Study the drawing (mm; zero at the part's minimum x, y, z) and answer. Give positions to 0.01 mm unless a question says otherwise; leave off trailing zeros. Write each loop counter-clockwise with the first axis right and the second up, starting at its lowest first coordinate (ties: lowest second). Pieces come first, ordered by that corner, then holes.
1) Find section C-C (z = 5). Determine the outline of the cut face in (x, y), plus the area to 3 significant figures.
2) Find section A-A (y = 10). Determine the outline of the cut face in (x, z), plus the area to 3 significant figures.
3) Straight lines are drawn through the part: probe 1 along Y at (x, z) = (10, 21); probe 2 along Z at (x, y) = (8.5, 12.5); probe 3 along X at (y, z) = (7.5, 43). For each, find the intervals that lie inside material, in ascending order.
4) Given pin 1 Ø8 at (x, z) = (6.5, 57) entering from +Y; pin 2 Ø6 at (y, z) = (12, 23) entering from +X; pin 3 Ø5.5 at (x, y) = (10, 10) entering from -Z, each flat-ended and moving along its own axis, determine where each tip first touches the part or whether it passes through.
5) Find section D-D (z = 15). Determine the outline of the cut face in (x, y), plus the area to 3 significant figures.
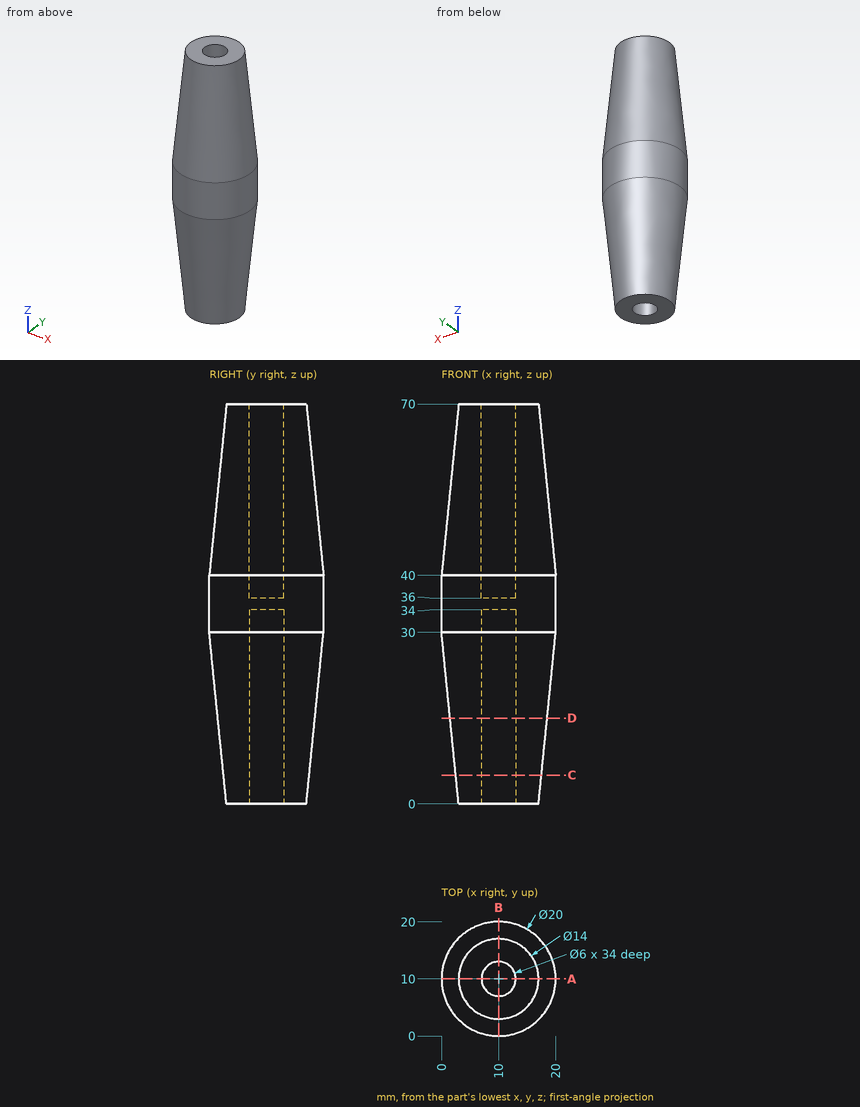
Results:
1. outline: circle Ø15 at (10, 10); hole circle Ø6 at (10, 10)
1. area: 148 mm2
2. outline: (0, 30) - (3, 0) - (7, 0) - (7, 34) - (13, 34) - (13, 0) - (17, 0) - (20, 30) - (20, 40) - (17, 70) - (13, 70) - (13, 36) - (7, 36) - (7, 70) - (3, 70) - (0, 40) - close
2. area: 812 mm2
3. probe 1: y = 0.9 to 7, 13 to 19.1
3. probe 2: z = 34 to 36
3. probe 3: x = 0.63 to 8.34, 11.66 to 19.37
4. pin 1: stops at y = 18.56
4. pin 2: stops at x = 19.55
4. pin 3: stops at z = 34
5. outline: circle Ø17 at (10, 10); hole circle Ø6 at (10, 10)
5. area: 199 mm2
